Input: dimensioned drawing with shaded views. Units: mm. Origin: part minimum x, y, z. A direction names the side the tool comes from. Coordinates: 2 decimals unless noted, no trailing zeros. Loops run counter-clockwise (first coordinate to the right, second up) from the corner with the lowest first, then second, coordinate; pieces in that order, holes last. Notation, with made-up numbers: (4.25, -27.5) - (62.25, -27.5) arc R27 cw to (62.25, -9.5) - close; hole circle Ø5 at (54, 78). An arc over 180 degrees is marked (long way). Write item = value, one per line. Start each with the question number.
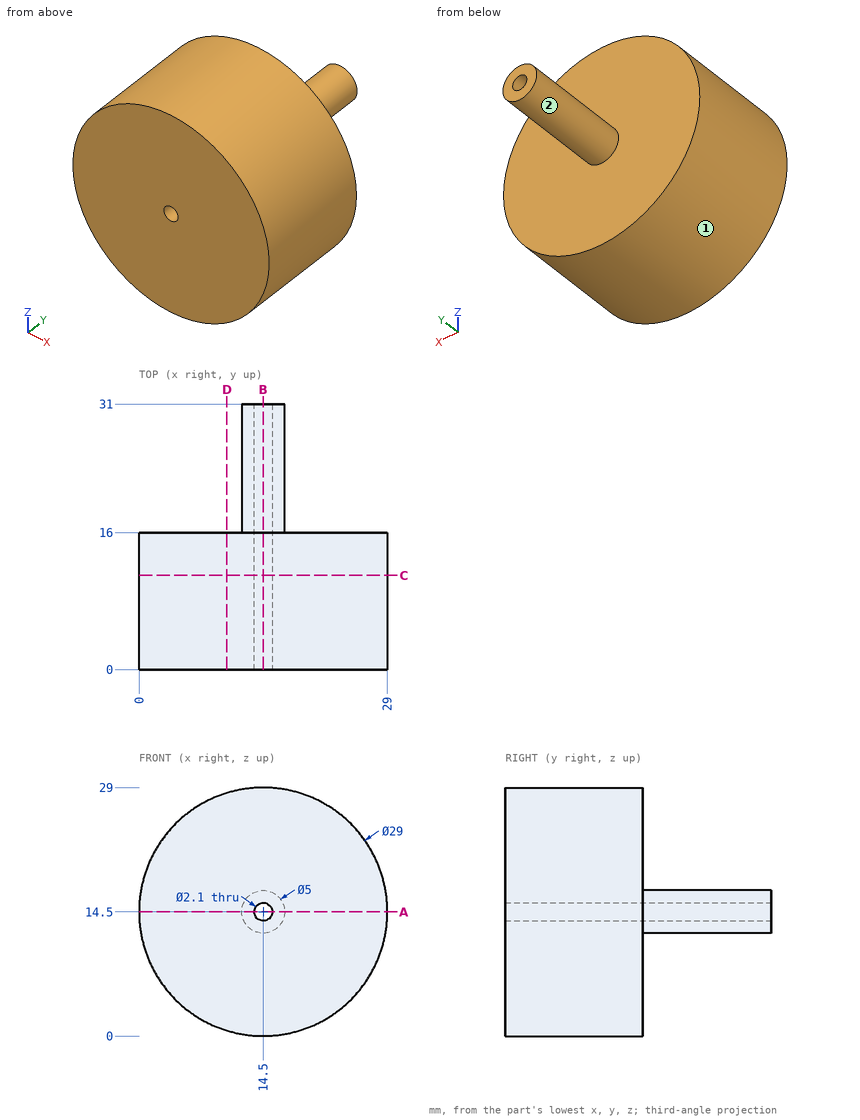
Item 1: Cut plane D-D on x = 10.25. Return loops of the section in (y, z).
Item 2: Pin query (flat end, axial travel): pin 1 (5 mm diameter, centred on y = 7.5, z = 3, fed in from -X); pin 2 (6 mm diameter, centred on x = 16, y = 21, fed in from +Z); pin 3 (6 mm diameter, centred on x = 11, y = 21, fed in from -Z). Return the tip coordinate at first contact, or that it passes through.
Item 3: Cut plane C-C on y = 11. Return loops of the section in (x, z).
Item 4: Ray query, line 1 (X direction, y = 21.5, z = 14.5); line 2 (Z direction, x = 14.5, y = 10.5). Return the intervals inside material, ascending.
Item 5: Cut plane A-A on z = 14.5. Return loops of the section in (x, y).
Item 6: Access query for the marked faces 1 and 2. Directions: +Z, -Z, +X, -X, +Y, -Y. A direction counts if a zero-diameter tool reaches every point of the face in a straight line with its end or side. Return the directions, or none.
Item 7: Cut plane B-B on x = 14.5. Return loops of the section in (y, z), plus the area to 3 significant figures.
Recorded:
q1.outline = (0, 0.64) - (16, 0.64) - (16, 28.36) - (0, 28.36) - close
q2.pin_1 = 3.13
q2.pin_2 = 17
q2.pin_3 = 12.05
q3.outline = circle Ø29 at (14.5, 14.5); hole circle Ø2.1 at (14.5, 14.5)
q4.line_1 = 12 to 13.45, 15.55 to 17
q4.line_2 = 0 to 13.45, 15.55 to 29
q5.outline = (0, 0) - (13.45, 0) - (13.45, 31) - (12, 31) - (12, 16) - (0, 16) - close; (15.55, 0) - (29, 0) - (29, 16) - (17, 16) - (17, 31) - (15.55, 31) - close
q6.face_1 = +Y, -Y
q6.face_2 = +Y
q7.outline = (0, 0) - (16, 0) - (16, 12) - (31, 12) - (31, 13.45) - (0, 13.45) - close; (0, 15.55) - (31, 15.55) - (31, 17) - (16, 17) - (16, 29) - (0, 29) - close
q7.area = 474 mm²
